```python
from build123d import *

# Parameters (mm, degrees)
SKETCH2_W           = 30
SKETCH2_H           = 20
BOSS_EXTRUDE2_DEPTH = 5
SKETCH3_R           = 5
BOSS_EXTRUDE3_DEPTH = 2
REVOLVE1_ANGLE      = 180
SKETCH5_R           = 0.625
CUT_EXTRUDE2_DEPTH  = 20


with BuildPart() as part:
    # Sketch2 → Boss-Extrude2 (new body)
    with BuildSketch(Plane(origin=(0, 0, 0), x_dir=(1, 0, 0), z_dir=(0, 1, 0))):
        with Locations((-3.934911243, 0.236686391)):
            Rectangle(SKETCH2_W, SKETCH2_H)
    extrude(amount=BOSS_EXTRUDE2_DEPTH)

    # Sketch3 → Boss-Extrude3 (add)
    with BuildSketch(Plane.XZ):
        with Locations(Location((-3.934911243, -0.236686391, 0), (0, 0, 270))):
            Circle(SKETCH3_R)
    extrude(amount=BOSS_EXTRUDE3_DEPTH)

    # Sketch4 → Revolve1 (revolve)
    with BuildSketch(Plane(origin=(0, -2, 0), x_dir=(-1, 0, 0), z_dir=(0, -1, 0))):
        with BuildLine():
            Line((3.934911243, -7.263313609), (3.934911243, 7.736686391))
            ThreePointArc((3.934911243, 7.736686391), (11.434911243, 0.236686391), (3.934911243, -7.263313609))
        make_face()
    revolve(axis=Axis((-3.934911243, -2, 7.263313609), (0, 0, 1)), revolution_arc=REVOLVE1_ANGLE)

    # Sketch5 → Cut-Extrude2 (cut)
    with BuildSketch(Plane.XY.offset(9.763313609)):
        with Locations((-12.684911243, 2.5)):
            Circle(SKETCH5_R)
        with Locations((4.815088757, 2.5)):
            Circle(SKETCH5_R)
    extrude(amount=-CUT_EXTRUDE2_DEPTH, mode=Mode.SUBTRACT)


solid = part.part
```
Geometry: final body of the model. Coordinates: model frame, mm. A direction names the side the tool comes from. Coordinates: 2 decimals unless noted, no trailing zeros. Order: outer loops, then holes, each group sorted by start corner. A loop starts at its lowest first (then second) coordinate and runs counter-clockwise, first axis right, second up. Notation, with made-up numbers: (67, 45.5) - (84, 45.5) arc R8 ccw to (84, 50.5) - close; hole circle Ø9 at (0, -3). An arc over 180 degrees is marked (long way). Return JSON: item names as keys, results as strings. Group by question number.
1. Pull-direction query (Y, two-part tool) for faces 1 (the face through (1, -2, 1.3)), 2 (the face through (-4, 2, -10.237)), 3 (the face through (-4, 5, 0)); classes: pulls with the +Y half, pulls with the -Y half, needs draft (parallel to the pull), parting line crosses it, or undercut.
2. Cut plane C-C (x = -1.75). Output: boundary loops of the cut face in (y, z).
3. Cut plane D-D (z = -3.75). Output: boundary loops of the cut face in (x, y) (3 decimals).
4. Cut plane B-B (z = 2). Output: boundary loops of the cut face in (x, y) (3 decimals).
5. Material intervals for line 1 along X through (y, z) = (2.75, -2.75); line 2 along Z through (x, y) = (-3.75, -1); line 3 along Y through (x, z) = (6.75, -2.5), sorted ascending. Write a range as [from, to].
6. Set-up query: faces 4 (the face through (-8.816, -0.986, 0.847)), 5 (the face through (11.065, 2, 0)). Return all of +Z, -Z, +X, -X, +Y, -Y with unobstructed straight access to the full face (end or side cutting, diameter ignored); none if empty.
7. Cut plane A-A (y = 2.5). Output: boundary loops of the cut face in (x, z), plus the area to 3 significant figures.
8. Pin query (flat end, axial travel): pin 1 (8 mm diameter, centred on x = 7.5, z = -7.5, fed in from -Y); pin 2 (4 mm diameter, centred on x = -1.5, z = 2.5, fed in from -Y); pin 3 (8 mm diameter, centred on y = -5, z = -7, fed in from +X); pin 4 (1.5 mm diameter, centred on x = -10.5, y = -1, fed in from +Z). Return the tip coordinate at first contact, or that it passes through.
Resolved:
{
 "1": {"face 1": "undercut", "face 2": "needs draft", "face 3": "pulls with the +Y half"},
 "2": {"outline": "(-2, -7.41) - (-2, -4.73) - (0, -4.73) - (0, -10.24) - (5, -10.24) - (5, 9.76) - (0, 9.76) - (0, 4.26) - (-2, 4.26) - (-2, 6.94) arc R7.17 ccw to start"},
 "3": {"outline": "(-18.935, 0) - (-7.493, 0) - (-7.493, -2) - (-10.561, -2) arc R6.626 ccw to (2.691, -2) - (-0.377, -2) - (-0.377, 0) - (11.065, 0) - (11.065, 5) - (-18.935, 5) - close; hole circle Ø1.25 at (-12.685, 2.5); hole circle Ø1.25 at (4.815, 2.5)"},
 "4": {"outline": "(-18.935, 0) - (-8.407, 0) - (-8.407, -2) - (-11.094, -2) arc R7.159 ccw to (3.224, -2) - (0.537, -2) - (0.537, 0) - (11.065, 0) - (11.065, 5) - (-18.935, 5) - close; hole circle Ø1.25 at (-12.685, 2.5); hole circle Ø1.25 at (4.815, 2.5)"},
 "5": {"line 1": "x = [-18.93, -13.26], [-12.11, 4.24], [5.39, 11.07]", "line 2": "z = [-5.23, 4.76]", "line 3": "y = [0, 5]"},
 "6": {"face 4": "none", "face 5": "+Z, -Z, +X, +Y, -Y"},
 "7": {"outline": "(-18.93, -10.24) - (-13.31, -10.24) - (-13.31, 9.76) - (-18.93, 9.76) - close; (-12.06, -10.24) - (4.19, -10.24) - (4.19, 9.76) - (-12.06, 9.76) - close; (5.44, -10.24) - (11.07, -10.24) - (11.07, 9.76) - (5.44, 9.76) - close", "area": "550 mm²"},
 "8": {"pin 1": "stops at y = 0", "pin 2": "stops at y = -9.31", "pin 3": "stops at x = 2.75", "pin 4": "passes through"}
}
